from build123d import *

# Parameters (mm, degrees)
SKETCH1_W           = 100
SKETCH1_H           = 55
SKETCH1_W_2         = 97.5
SKETCH1_H_2         = 52.5
BOSS_EXTRUDE1_DEPTH = 2
FILLET1_R           = 1.5


with BuildPart() as part:
    # Sketch1 → Boss-Extrude1 (new body)
    with BuildSketch(Plane.XY):
        with Locations((12.10302883, 11.151503687)):
            Rectangle(SKETCH1_W, SKETCH1_H)
        with Locations((12.10302883, 11.151503687)):
            Rectangle(SKETCH1_W_2, SKETCH1_H_2, mode=Mode.SUBTRACT)
    extrude(amount=BOSS_EXTRUDE1_DEPTH)

    # Fillet1
    fillet1_edges = [part.edges().sort_by_distance(p)[0] for p in [
        (-37.89697117, 38.651503687, 1),
        (62.10302883, 38.651503687, 1),
        (62.10302883, -16.348496313, 1),
        (-37.89697117, -16.348496313, 1),
    ]]
    fillet(fillet1_edges, radius=FILLET1_R)


solid = part.part
The model under review builds one solid part; all positions refer to its coordinate system, in mm. A direction names the side the tool comes from. Coordinates: 2 decimals unless noted, no trailing zeros. Write each loop counter-clockwise with the first axis right and the second up, starting at its lowest first coordinate (ties: lowest second). Pieces come first, ordered by that corner, then holes. Notation, with made-up numbers: (81.25, -18) - (89.25, -18) arc R11 cw to (89.25, -1) - close; hole circle Ø7 at (-21, 29). An arc over 180 degrees is marked (long way). Answer as a JSON object with one key per item and string values. Group by question number.
1. Machinability: for faces 5 (the face through (62.103, 11, 1)), 6 (the face through (11, -15.098, 1)), which of the approach directions +Z, -Z, +X, -X, +Y, -Y give a long, thin tool a straight path to every point of the face, cutting with its end or side? Answer none if there is none.
2. Add section B-B (x = -7.5). Give the boundary of the cut face in (y, z), plus the area to 3 significant figures.
3. To check wall thickness, follow probe 1 along X at (y, z) = (12, 1.95); probe 2 along Y at (x, z) = (-18, 0.8). State the ranges of each line that lie inside material, in increasing order.
4. Mouldability with a two-part tool opening along Y and no side actions: class faces 1 (the face through (11, 38.652, 1)), 2 (the face through (-37.897, 11, 1)), 3 (the face through (11, -16.348, 1)), 4 (the face through (-36.647, 11, 1)) as pulls with the +Y half, pulls with the -Y half, needs draft (parallel to the pull), parting line crosses it, or undercut.
5. Add section C-C (z = 0.9). Give the boundary of the cut face in (x, y), plus the area to 3 significant figures.
6. Add section A-A (y = -2). Give the boundary of the cut face in (x, z).
Findings:
{
 "1": {"face 5": "+Z, -Z, +X, +Y, -Y", "face 6": "+Z, -Z"},
 "2": {"outline": "(-16.35, 0) - (-15.1, 0) - (-15.1, 2) - (-16.35, 2) - close; (37.4, 0) - (38.65, 0) - (38.65, 2) - (37.4, 2) - close", "area": "5.00 mm²"},
 "3": {"probe 1": "-37.9 to -36.65, 60.85 to 62.1", "probe 2": "-16.35 to -15.1, 37.4 to 38.65"},
 "4": {"face 1": "pulls with the +Y half", "face 2": "needs draft", "face 3": "pulls with the -Y half", "face 4": "undercut"},
 "5": {"outline": "(-37.9, -14.85) arc R1.5 ccw to (-36.4, -16.35) - (60.6, -16.35) arc R1.5 ccw to (62.1, -14.85) - (62.1, 37.15) arc R1.5 ccw to (60.6, 38.65) - (-36.4, 38.65) arc R1.5 ccw to (-37.9, 37.15) - close; hole (-36.65, -15.1) - (60.85, -15.1) - (60.85, 37.4) - (-36.65, 37.4) - close", "area": "379 mm²"},
 "6": {"outline": "(-37.9, 0) - (-36.65, 0) - (-36.65, 2) - (-37.9, 2) - close; (60.85, 0) - (62.1, 0) - (62.1, 2) - (60.85, 2) - close"}
}
